CAD build for the part. Positions are in the model's coordinates, mm. A direction names the side the tool comes from. Round coordinates to 2 decimals unless told otherwise and drop trailing zeros. Order: outer loops, then holes, each group sorted by start corner. A loop starts at its lowest first (then second) coordinate and runs counter-clockwise, first axis right, second up. Notation, with made-up numbers: (69, 58.5) - (88, 58.5) arc R14 cw to (88, 73.5) - close; hole circle Ø2 at (3, 31.25). An arc over 180 degrees is marked (long way). Write item = value, one per line.
from build123d import *

# Parameters (mm, degrees)
F0_W     = 76.2
F0_H     = 152.4
F0_W_2   = 66.675
F0_H_2   = 142.875
F0_R     = 3.1
F1_DEPTH = 4.7625
F2_DEPTH = 31.75
F3_DEPTH = 25.4
F4_DEPTH = 4.7625


with BuildPart() as f1:
    # F0 (on Top) → F1 (new body)
    with BuildSketch(Plane.XY):
        with Locations((3.610619, 24.259033)):
            Rectangle(F0_W, F0_H)
        with Locations((3.610619, 24.259033)):
            Rectangle(F0_W_2, F0_H_2, mode=Mode.SUBTRACT)
        with Locations((3.610619, 24.259033)):
            Rectangle(F0_W_2, F0_H_2)
        with BuildLine():
            ThreePointArc((-28.464381, 36.084033), (-27.585701, 38.205353), (-25.464381, 39.084033))
            Line((-25.464381, 39.084033), (24.535619, 39.084033))
            ThreePointArc((24.535619, 39.084033), (26.65694, 38.205353), (27.535619, 36.084033))
            Line((27.535619, 36.084033), (27.535619, -42.915967))
            ThreePointArc((27.535619, -42.915967), (26.65694, -45.037288), (24.535619, -45.915967))
            Line((24.535619, -45.915967), (-25.464381, -45.915967))
            ThreePointArc((-25.464381, -45.915967), (-27.585701, -45.037288), (-28.464381, -42.915967))
            Line((-28.464381, -42.915967), (-28.464381, 36.084033))
        make_face(mode=Mode.SUBTRACT)
        with BuildLine():
            Line((24.535619, 39.084033), (-25.464381, 39.084033))
            ThreePointArc((-25.464381, 39.084033), (-27.585701, 38.205353), (-28.464381, 36.084033))
            Line((-28.464381, 36.084033), (-28.464381, -42.915967))
            ThreePointArc((-28.464381, -42.915967), (-27.585701, -45.037288), (-25.464381, -45.915967))
            Line((-25.464381, -45.915967), (24.535619, -45.915967))
            ThreePointArc((24.535619, -45.915967), (26.65694, -45.037288), (27.535619, -42.915967))
            Line((27.535619, -42.915967), (27.535619, 36.084033))
            ThreePointArc((27.535619, 36.084033), (26.65694, 38.205353), (24.535619, 39.084033))
        make_face()
        with Locations((-24.964381, -42.415967)):
            Circle(F0_R, mode=Mode.SUBTRACT)
        with Locations((-24.964381, 15.584033)):
            Circle(F0_R, mode=Mode.SUBTRACT)
        with Locations((24.035619, -42.415967)):
            Circle(F0_R, mode=Mode.SUBTRACT)
        with Locations((24.035619, 15.584033)):
            Circle(F0_R, mode=Mode.SUBTRACT)
        with Locations((24.035619, 15.584033)):
            Circle(F0_R)
        with Locations((24.035619, -42.415967)):
            Circle(F0_R)
        with Locations((-24.964381, -42.415967)):
            Circle(F0_R)
        with Locations((-24.964381, 15.584033)):
            Circle(F0_R)
    extrude(amount=-F1_DEPTH)

    # F0 (on Top) → F2 (join)
    with BuildSketch(Plane.XY):
        with Locations((3.610619, 24.259033)):
            Rectangle(F0_W, F0_H)
        with Locations((3.610619, 24.259033)):
            Rectangle(F0_W_2, F0_H_2, mode=Mode.SUBTRACT)
    extrude(amount=F2_DEPTH)

    # F0 (on Top) → F3 (join)
    with BuildSketch(Plane.XY):
        with Locations((3.610619, 24.259033)):
            Rectangle(F0_W, F0_H)
        with Locations((3.610619, 24.259033)):
            Rectangle(F0_W_2, F0_H_2, mode=Mode.SUBTRACT)
    extrude(amount=F3_DEPTH)

    # F0 (on Top) → F4 (join)
    with BuildSketch(Plane.XY):
        with Locations((24.035619, 15.584033)):
            Circle(F0_R)
        with Locations((24.035619, -42.415967)):
            Circle(F0_R)
        with Locations((-24.964381, -42.415967)):
            Circle(F0_R)
        with Locations((-24.964381, 15.584033)):
            Circle(F0_R)
    extrude(amount=F4_DEPTH)


solid = f1.part
(1) Band-saw the part on A-A on z = 1.5. List the corners of the cut face in (x, y).
Solved:
outline = (-34.49, -51.94) - (41.71, -51.94) - (41.71, 100.46) - (-34.49, 100.46) - close; circle Ø6.2 at (-24.96, -42.42); circle Ø6.2 at (-24.96, 15.58); circle Ø6.2 at (24.04, -42.42); circle Ø6.2 at (24.04, 15.58); hole (-29.73, -47.18) - (36.95, -47.18) - (36.95, 95.7) - (-29.73, 95.7) - close
(2) Band-saw the part on C-C on y = 69.5. List the corners of the cut face in (x, z).
Solved:
outline = (-34.49, -4.76) - (41.71, -4.76) - (41.71, 31.75) - (36.95, 31.75) - (36.95, 0) - (-29.73, 0) - (-29.73, 31.75) - (-34.49, 31.75) - close
(3) Drop flat-ended pins along their axis: pin 1 (3 mm diameter, centred on x = -26, y = 14, fed in from +Z); pin 2 (6 mm diameter, centred on x = 28, y = -22, fed in from +Z). Give the stop position or say it passes through.
Solved:
pin_1 = 4.76
pin_2 = 0
(4) Tool access for faces 1 (the flat face through (-25, -42, 4.762)), 2 (the flat face through (3, -51.941, 13)): list every direction of +Z, -Z, +X, -X, +Y, -Y with a clear straight run to the whole face (end or side of a thin tool).
Solved:
face_1 = +Z
face_2 = +Z, -Z, +X, -X, -Y
(5) Band-saw the part on D-D on x = 22.5. List the corners of the cut face in (y, z), plus the area to 3 significant figures.
Solved:
outline = (-51.94, -4.76) - (100.46, -4.76) - (100.46, 31.75) - (95.7, 31.75) - (95.7, 0) - (18.28, 0) - (18.28, 4.76) - (12.89, 4.76) - (12.89, 0) - (-39.72, 0) - (-39.72, 4.76) - (-45.11, 4.76) - (-45.11, 0) - (-47.18, 0) - (-47.18, 31.75) - (-51.94, 31.75) - close
area = 1,080 mm²
(6) Band-saw the part on B-B on x = 34.5. List the corners of the cut face in (y, z).
Solved:
outline = (-51.94, -4.76) - (100.46, -4.76) - (100.46, 31.75) - (95.7, 31.75) - (95.7, 0) - (-47.18, 0) - (-47.18, 31.75) - (-51.94, 31.75) - close
(7) Pull direction X, two halves, no side cores. Call faces 3 (the flat face through (3, 100.459, 13)), 4 (the flat face through (-34.489, 23, 13)), 5 (the flat face through (3, 95.697, 16)): released by +X, released by -X, zero draft, split by the parting line, or undercut.
Solved:
face_3 = zero draft
face_4 = released by -X
face_5 = undercut
(8) Probe line 1 along X through (y, z) = (-40.5, 12.5); line 2 along Y through (x, z) = (-15.5, 10.5); line 3 along Y through (x, z) = (26.5, 3.5). List the from-to ranges inside material, lowest first.
Solved:
line_1 = -34.49 to -29.73, 36.95 to 41.71
line_2 = -51.94 to -47.18, 95.7 to 100.46
line_3 = -51.94 to -47.18, -44.3 to -40.54, 13.7 to 17.46, 95.7 to 100.46
